Work out the finished part from the listing and answer in its coordinate system (mm). A direction names the side the tool comes from. Give positions to 0.01 mm unless a question says otherwise; leave off trailing zeros. Loops run counter-clockwise (first coordinate to the right, second up) from the corner with the lowest first, then second, coordinate; pieces in that order, holes last. Notation, with made-up numbers: (-16.75, -3.75) - (38.25, -3.75) arc R17 cw to (38.25, 10.25) - close; hole circle Ø2 at (82.25, 34.5). An arc over 180 degrees is marked (long way). One line per item, written item: value.
from build123d import *

# Parameters (mm, degrees)
RECTANGLE077_W         = 0.2
RECTANGLE077_H         = 33.4
EXTRUDE207_DEPTH       = 1.5
RECTANGLE072_W         = 32.9
RECTANGLE072_H         = 33.4
EXTRUDE172_DEPTH       = 0.5
CIRCLE037_R            = 0.6
EXTRUDE166_DEPTH       = 2.8
CIRCLE036_R            = 0.6
EXTRUDE163_DEPTH       = 2.8
CIRCLE038_R            = 0.6
EXTRUDE165_DEPTH       = 2.8
CIRCLE040_R            = 0.65
EXTRUDE167_DEPTH       = 10
CIRCLE018_R            = 2
EXTRUDE155_DEPTH       = 2.1
RECTANGLE065_W         = 2
RECTANGLE065_H         = 1
EXTRUDE156_DEPTH       = 2.1
RECTANGLE064_W         = 2
RECTANGLE064_H         = 1
EXTRUDE153_DEPTH       = 2.1
CIRCLE019_R            = 2
EXTRUDE152_DEPTH       = 2.1
RECTANGLE066_W         = 1
RECTANGLE066_H         = 1
EXTRUDE150_DEPTH       = 2.1
CIRCLE020_R            = 2
EXTRUDE149_DEPTH       = 2.1
RECTANGLE070_W         = 7.6
RECTANGLE070_H         = 23
EXTRUDE162_DEPTH       = 2.8
RECTANGLE061_W         = 24.1
RECTANGLE061_H         = 25.1
EXTRUDE117_DEPTH       = 6.2
RECTANGLE063_W         = 1.5
RECTANGLE063_H         = 23
EXTRUDE128_DEPTH       = 8
RECTANGLE060_W         = 14.4
RECTANGLE060_H         = 23
EXTRUDE141_DEPTH       = 8
RECTANGLE059_W         = 15.5
RECTANGLE059_H         = 19
EXTRUDE140_DEPTH       = 8
RECTANGLE062_W         = 29.9
RECTANGLE062_H         = 30.4
EXTRUDE116_DEPTH       = 5
RECTANGLE053_W         = 32.9
RECTANGLE053_H         = 33.4
EXTRUDE107_DEPTH       = 9
RECTANGLE067_W         = 1
RECTANGLE067_H         = 1
EXTRUDE159_DEPTH       = 2.1
CIRCLE021_R            = 2
EXTRUDE158_DEPTH       = 2.1
CUT078_PLACEMENT_ANGLE = 180


with BuildPart() as extrude207:
    # Rectangle077 → Extrude207 (new body)
    with BuildSketch(Plane(origin=(50.534308, -80.765974, -19.3), x_dir=(1, 0, 0), z_dir=(0, 0, 1))):
        with Locations((0.1, 16.7)):
            Rectangle(RECTANGLE077_W, RECTANGLE077_H)
    extrude(amount=EXTRUDE207_DEPTH)


with BuildPart() as extrude172:
    # Rectangle072 (on Cut) → Extrude172 (new body)
    with BuildSketch(Plane(origin=(17.834308, -47.365974, -18.8), x_dir=(1, 0, 0), z_dir=(0, 0, -1))):
        with Locations((16.45, 16.7)):
            Rectangle(RECTANGLE072_W, RECTANGLE072_H)
    extrude(amount=EXTRUDE172_DEPTH)


with BuildPart() as extrude166:
    # Circle037 → Extrude166 (new body)
    with BuildSketch(Plane(origin=(67.748726, -53.60327, -3.6), x_dir=(1, 0, 0), z_dir=(0, 0, -1))):
        Circle(CIRCLE037_R)
    extrude(amount=-EXTRUDE166_DEPTH)


with BuildPart() as extrude163:
    # Circle036 → Extrude163 (new body)
    with BuildSketch(Plane(origin=(80.134308, -53.565974, -3.6), x_dir=(1, 0, 0), z_dir=(0, 0, 1))):
        Circle(CIRCLE036_R)
    extrude(amount=EXTRUDE163_DEPTH)


with BuildPart() as extrude165:
    # Circle038 → Extrude165 (new body)
    with BuildSketch(Plane(origin=(67.634308, -74.565974, -3.6), x_dir=(1, 0, 0), z_dir=(0, 0, 1))):
        Circle(CIRCLE038_R)
    extrude(amount=EXTRUDE165_DEPTH)


with BuildPart() as extrude167:
    # Circle040 (on Cut) → Extrude167 (new body)
    with BuildSketch(Plane(origin=(80.134308, -74.565974, -3.6), x_dir=(1, 0, 0), z_dir=(0, 0, -1))):
        Circle(CIRCLE040_R)
    extrude(amount=-EXTRUDE167_DEPTH)


with BuildPart() as extrude155:
    # Circle018 → Extrude155 (new body)
    with BuildSketch(Plane(origin=(80.134308, -53.565974, -3.6), x_dir=(1, 0, 0), z_dir=(0, 0, 1))):
        Circle(CIRCLE018_R)
    extrude(amount=EXTRUDE155_DEPTH)


with BuildPart() as fusion026:
    # Rectangle065 → Extrude156 (new body)
    with BuildSketch(Plane(origin=(80.134308, -55.565974, -3.6), x_dir=(1, 0, 0), z_dir=(0, 0, 1))):
        with Locations((1, 0.5)):
            Rectangle(RECTANGLE065_W, RECTANGLE065_H)
    extrude(amount=EXTRUDE156_DEPTH)

    # Fusion026: union Extrude155
    add(extrude155.part)


with BuildPart() as extrude153:
    # Rectangle064 → Extrude153 (new body)
    with BuildSketch(Plane(origin=(80.134308, -73.565974, -3.6), x_dir=(1, 0, 0), z_dir=(0, 0, 1))):
        with Locations((1, 0.5)):
            Rectangle(RECTANGLE064_W, RECTANGLE064_H)
    extrude(amount=EXTRUDE153_DEPTH)


with BuildPart() as fusion032:
    # Circle019 → Extrude152 (new body)
    with BuildSketch(Plane(origin=(80.134308, -74.565974, -3.6), x_dir=(1, 0, 0), z_dir=(0, 0, 1))):
        Circle(CIRCLE019_R)
    extrude(amount=EXTRUDE152_DEPTH)

    # Fusion032: union Extrude153
    add(extrude153.part)


with BuildPart() as extrude150:
    # Rectangle066 → Extrude150 (new body)
    with BuildSketch(Plane(origin=(65.634308, -75.565974, -3.6), x_dir=(1, 0, 0), z_dir=(0, 0, 1))):
        with Locations((0.5, 0.5)):
            Rectangle(RECTANGLE066_W, RECTANGLE066_H)
    extrude(amount=EXTRUDE150_DEPTH)


with BuildPart() as fusion024:
    # Circle020 → Extrude149 (new body)
    with BuildSketch(Plane(origin=(67.634308, -74.565974, -3.6), x_dir=(1, 0, 0), z_dir=(0, 0, 1))):
        Circle(CIRCLE020_R)
    extrude(amount=EXTRUDE149_DEPTH)

    # Fusion024: union Extrude150
    add(extrude150.part)


with BuildPart() as extrude162:
    # Rectangle070 → Extrude162 (new body)
    with BuildSketch(Plane(origin=(58.034308, -75.565974, -3.6), x_dir=(1, 0, 0), z_dir=(0, 0, 1))):
        with Locations((3.8, 11.5)):
            Rectangle(RECTANGLE070_W, RECTANGLE070_H)
    extrude(amount=EXTRUDE162_DEPTH)


with BuildPart() as extrude117:
    # Rectangle061 → Extrude117 (new body)
    with BuildSketch(Plane(origin=(58.034308, -51.515974, -9.8), x_dir=(1, 0, 0), z_dir=(0, 0, -1))):
        with Locations((12.05, 12.55)):
            Rectangle(RECTANGLE061_W, RECTANGLE061_H)
    extrude(amount=-EXTRUDE117_DEPTH)


with BuildPart() as extrude128:
    # Rectangle063 → Extrude128 (new body)
    with BuildSketch(Plane(origin=(50.734308, -75.565974, -9.8), x_dir=(1, 0, 0), z_dir=(0, 0, 1))):
        with Locations((0.75, 11.5)):
            Rectangle(RECTANGLE063_W, RECTANGLE063_H)
    extrude(amount=EXTRUDE128_DEPTH)


with BuildPart() as extrude141:
    # Rectangle060 → Extrude141 (new body)
    with BuildSketch(Plane(origin=(52.234308, -52.565974, -9.8), x_dir=(1, 0, 0), z_dir=(0, 0, -1))):
        with Locations((7.2, 11.5)):
            Rectangle(RECTANGLE060_W, RECTANGLE060_H)
    extrude(amount=-EXTRUDE141_DEPTH)


with BuildPart() as extrude140:
    # Rectangle059 → Extrude140 (new body)
    with BuildSketch(Plane(origin=(66.634308, -54.565974, -9.8), x_dir=(1, 0, 0), z_dir=(0, 0, -1))):
        with Locations((7.75, 9.5)):
            Rectangle(RECTANGLE059_W, RECTANGLE059_H)
    extrude(amount=-EXTRUDE140_DEPTH)


with BuildPart() as extrude116:
    # Rectangle062 → Extrude116 (new body)
    with BuildSketch(Plane(origin=(52.234308, -48.865974, -9.8), x_dir=(1, 0, 0), z_dir=(0, 0, -1))):
        with Locations((14.95, 15.2)):
            Rectangle(RECTANGLE062_W, RECTANGLE062_H)
    extrude(amount=-EXTRUDE116_DEPTH)


with BuildPart() as cut074:
    # Rectangle053 → Extrude107 (new body)
    with BuildSketch(Plane(origin=(50.734308, -47.365974, -9.8), x_dir=(1, 0, 0), z_dir=(0, 0, -1))):
        with Locations((16.45, 16.7)):
            Rectangle(RECTANGLE053_W, RECTANGLE053_H)
    extrude(amount=-EXTRUDE107_DEPTH)

    # Cut046: cut Extrude116
    add(extrude116.part, mode=Mode.SUBTRACT)

    # Cut060: cut Extrude140
    add(extrude140.part, mode=Mode.SUBTRACT)

    # Cut061: cut Extrude141
    add(extrude141.part, mode=Mode.SUBTRACT)

    # Cut062: cut Extrude128
    add(extrude128.part, mode=Mode.SUBTRACT)

    # Cut063: cut Extrude117
    add(extrude117.part, mode=Mode.SUBTRACT)

    # Cut074: cut Extrude162
    add(extrude162.part, mode=Mode.SUBTRACT)


with BuildPart() as extrude159:
    # Rectangle067 → Extrude159 (new body)
    with BuildSketch(Plane(origin=(65.634308, -53.565974, -3.6), x_dir=(1, 0, 0), z_dir=(0, 0, 1))):
        with Locations((0.5, 0.5)):
            Rectangle(RECTANGLE067_W, RECTANGLE067_H)
    extrude(amount=EXTRUDE159_DEPTH)


with BuildPart() as cut_lens_capsule:
    # Circle021 → Extrude158 (new body)
    with BuildSketch(Plane(origin=(67.634308, -53.565974, -3.6), x_dir=(1, 0, 0), z_dir=(0, 0, 1))):
        Circle(CIRCLE021_R)
    extrude(amount=EXTRUDE158_DEPTH)

    # Fusion025: union Extrude159
    add(extrude159.part)

    # Fusion033: union Fusion026, Fusion032, Fusion024, Cut074
    add(fusion026.part)
    add(fusion032.part)
    add(fusion024.part)
    add(cut074.part)

    # Cut075: cut Extrude167
    add(extrude167.part, mode=Mode.SUBTRACT)

    # Cut076: cut Extrude165
    add(extrude165.part, mode=Mode.SUBTRACT)

    # Cut077: cut Extrude163
    add(extrude163.part, mode=Mode.SUBTRACT)

    # Cut078: cut Extrude166
    add(extrude166.part, mode=Mode.SUBTRACT)


with BuildPart() as cut_lens_capsule_1:
    # Cut078 placement: moved
    add(cut_lens_capsule.part.moved(Location((101.468615, 0, -19.6))).rotate(Axis((101.468615, 0, -19.6), (0, 1, 0)), CUT078_PLACEMENT_ANGLE))

    # Fusion035: union Extrude172
    add(extrude172.part)

    # Cut108: cut Extrude207
    add(extrude207.part, mode=Mode.SUBTRACT)


solid = cut_lens_capsule_1.part
1. For faces 1 (the flat face through (47, -64, -17.8)), 2 (the flat face through (49.234, -51, -12)), 3 (the flat face through (50.534, -64, -19)), 4 (the flat face through (34, -64, -19.3)), determine the directions among +Z, -Z, +X, -X, +Y, -Y from which every point of the face is accessible in a straight line to the end or side of a thin tool.
Output:
face 1: +Z, +X
face 2: +Z
face 3: -Z, +X, +Y, -Y
face 4: -Z, +X, -X, +Y, -Y
2. Find the intervals of material crossed by line 1 along Y through (x, z) = (37, -12); line 2 along X through (y, z) = (-70, -18.25); line 3 along Y through (x, z) = (31.5, -17), in increasing order.
Output:
line 1: y = -80.77 to -79.27, -48.87 to -47.37
line 2: x = 17.83 to 35.83, 43.43 to 50.53
line 3: y = -80.77 to -73.57, -54.57 to -47.37
3. The mould has two halves that part along Y. Classify faces 5 (the flat face through (28, -64, -17.8)), 6 (the flat face through (32, -76.616, -15)), 7 (the flat face through (19, -64, -9.8)): released by +Y, released by -Y, zero draft, split by the parting line, or undercut.
Output:
face 5: undercut
face 6: undercut
face 7: zero draft
4. Section A-A (x = 29.5) is taken. Write down the section's boundary in (y, z), and give its area (3 significant figures).
Output:
outline: (-80.77, -19.3) - (-47.37, -19.3) - (-47.37, -9.8) - (-48.87, -9.8) - (-48.87, -14.8) - (-51.52, -14.8) - (-51.52, -16) - (-54.57, -16) - (-54.57, -17.8) - (-73.57, -17.8) - (-73.57, -16) - (-76.62, -16) - (-76.62, -14.8) - (-79.27, -14.8) - (-79.27, -9.8) - (-80.77, -9.8) - close
area: 101 mm²
5. Section C-C (z = -11.75) is taken. Write down the section's boundary in (x, y).
Output:
outline: (17.83, -80.77) - (50.73, -80.77) - (50.73, -75.57) - (49.23, -75.57) - (49.23, -79.27) - (19.33, -79.27) - (19.33, -48.87) - (49.23, -48.87) - (49.23, -52.57) - (50.73, -52.57) - (50.73, -47.37) - (17.83, -47.37) - close
6. Flat-ended cylindrical pins translate along their axes: pin 1 Ø2.5 at (x, y) = (39.5, -62.5) entering from +Z; pin 2 Ø4 at (x, y) = (35.5, -51) entering from +Z; pin 3 Ø2 at (y, z) = (-64.5, -17.5) entering from +X; pin 4 Ø4 at (y, z) = (-53.5, -18) entering from +X. Find the tip coordinate at first contact, or state that the pin passes through.
Output:
pin 1: stops at z = -18.8
pin 2: stops at z = -14.8
pin 3: stops at x = 50.53
pin 4: stops at x = 50.73
7. Section D-D (z = -17) is taken. Write down the section's boundary in (x, y), and give its area (3 significant figures).
Output:
outline: (17.83, -80.77) - (50.73, -80.77) - (50.73, -75.57) - (35.83, -75.57) - (35.83, -74.57) arc R2 ccw to (32.1, -73.57) - (23.07, -73.57) arc R2 ccw to (21.33, -72.57) - (19.33, -72.57) - (19.33, -55.57) - (21.33, -55.57) arc R2 ccw to (23.07, -54.57) - (32.1, -54.57) arc R2 ccw to (35.83, -53.57) - (35.83, -52.57) - (50.73, -52.57) - (50.73, -47.37) - (17.83, -47.37) - close; hole circle Ø1.3 at (21.33, -74.57); hole circle Ø1.2 at (21.33, -53.57); hole circle Ø1.2 at (33.72, -53.6); hole circle Ø1.2 at (33.83, -74.57)
area: 449 mm²
